from build123d import *

# Parameters (mm, degrees)
SKETCH001_W   = 34
SKETCH001_H   = 32
SKETCH001_R   = 2.5
SKETCH001_R_2 = 9
PAD001_DEPTH  = 2
FILLET_R      = 2


with BuildPart() as part:
    # Sketch001 → Pad001 (new body)
    with BuildSketch(Plane.XY):
        Rectangle(SKETCH001_W, SKETCH001_H)
        with Locations((-9.2, 10.5)):
            Circle(SKETCH001_R, mode=Mode.SUBTRACT)
        with Locations((9.2, 10.5)):
            Circle(SKETCH001_R, mode=Mode.SUBTRACT)
        with Locations((-9.2, -10.5)):
            Circle(SKETCH001_R, mode=Mode.SUBTRACT)
        with Locations((9.2, -10.5)):
            Circle(SKETCH001_R, mode=Mode.SUBTRACT)
        Circle(SKETCH001_R_2, mode=Mode.SUBTRACT)
    extrude(amount=-PAD001_DEPTH)

    # Fillet
    fillet_edges = [part.edges().sort_by_distance(p)[0] for p in [
        (17, -16, -1),
        (17, 16, -1),
        (-17, -16, -1),
        (-17, 16, -1),
    ]]
    fillet(fillet_edges, radius=FILLET_R)


solid = part.part
Verification items for the finished model (mm, model axes). Coordinates: 2 decimals unless noted, no trailing zeros. Loops run counter-clockwise (first coordinate to the right, second up) from the corner with the lowest first, then second, coordinate; pieces in that order, holes last. Notation, with made-up numbers: (83.5, -8) -> (111.5, -8) arc R23 cw to (111.5, 4) -> close; hole circle Ø1 at (-6.75, 15). An arc over 180 degrees is marked (long way). Write each question's results on one line, items separated by ' | '.
Item 1: Section check D-D, the plane y = 5.5. Enter the section's corners in (x, z), plus the area to 3 significant figures.
Found:
outline: (-17, -2) -> (-7.12, -2) -> (-7.12, 0) -> (-17, 0) -> close; (7.12, -2) -> (17, -2) -> (17, 0) -> (7.12, 0) -> close | area: 39.5 mm2
Item 2: Section check B-B, the plane y = 10.5. Enter the section's corners in (x, z).
Found:
outline: (-17, -2) -> (-11.7, -2) -> (-11.7, 0) -> (-17, 0) -> close; (-6.7, -2) -> (6.7, -2) -> (6.7, 0) -> (-6.7, 0) -> close; (11.7, -2) -> (17, -2) -> (17, 0) -> (11.7, 0) -> close
Item 3: Material ranges on L1, parallel to Y at x = -9.2, z = -1.25; L2, parallel to Y at x = 0, z = -0.8; L3, parallel to X at y = -11, z = -1.3, recorded low to high.
Found:
L1: y = -16 to -13, -8 to 8, 13 to 16 | L2: y = -16 to -9, 9 to 16 | L3: x = -17 to -11.65, -6.75 to 6.75, 11.65 to 17
Item 4: Gauge pin test, flat end, axial feed: pin 1 (4 mm diameter, centred on x = 9.2, y = -10.5, fed in from +Z). Record the tip position at first contact, or that the pin passes through.
Found:
pin 1: passes through
Item 5: Section check A-A, the plane z = -1.65. Enter the section's corners in (x, y), plus the area to 3 significant figures.
Found:
outline: (-17, -14) arc R2 ccw to (-15, -16) -> (15, -16) arc R2 ccw to (17, -14) -> (17, 14) arc R2 ccw to (15, 16) -> (-15, 16) arc R2 ccw to (-17, 14) -> close; hole circle Ø5 at (-9.2, -10.5); hole circle Ø5 at (-9.2, 10.5); hole circle Ø18 at (0, 0); hole circle Ø5 at (9.2, -10.5); hole circle Ø5 at (9.2, 10.5) | area: 752 mm2
Item 6: Mould release check, pull along Y, two halves, no side actions. Record for faces 1 (the face through (16.4, 15.43, -1.01)), 2 (the face through (10.35, -12.72, -0.99)), 3 (the face through (17, 0, -1)), 4 (the face through (16.4, -15.43, -1.01)): +Y half, -Y half, draft (parallel to the pull), parting line (faces both ways), or undercut.
Found:
face 1: +Y half | face 2: undercut | face 3: draft | face 4: -Y half
Item 7: Section check C-C, the plane x = 0. Enter the section's corners in (y, z).
Found:
outline: (-16, -2) -> (-9, -2) -> (-9, 0) -> (-16, 0) -> close; (9, -2) -> (16, -2) -> (16, 0) -> (9, 0) -> close
